```python
from build123d import *

# Parameters (mm, degrees)
BOSS_EXTRUDE1_DEPTH                               = 75
SKETCH5_R                                         = 1.75
CUT_EXTRUDE1_DEPTH                                = 2
CSK_FOR_0_FLAT_HEAD_MACHINE_SCREW_100_D           = 1.778
CSK_FOR_0_FLAT_HEAD_MACHINE_SCREW_100_DEPTH       = 3.302
CSK_FOR_0_FLAT_HEAD_MACHINE_SCREW_100_CSINK_D     = 3.0226
CSK_FOR_0_FLAT_HEAD_MACHINE_SCREW_100_CSINK_ANGLE = 100
CSK_FOR_0_FLAT_HEAD_MACHINE_SCREW_100_TIP         = 0.53416509
CHAMFER1_SIZE                                     = 3
BOSS_EXTRUDE2_DEPTH                               = 5
CHAMFER2_SIZE                                     = 3
CSK_FOR_0_FLAT_HEAD_MACHINE_SCREW_2_D             = 1.778
CSK_FOR_0_FLAT_HEAD_MACHINE_SCREW_2_DEPTH         = 3.302
CSK_FOR_0_FLAT_HEAD_MACHINE_SCREW_2_CSINK_D       = 3.0226
CSK_FOR_0_FLAT_HEAD_MACHINE_SCREW_2_CSINK_ANGLE   = 100
CSK_FOR_0_FLAT_HEAD_MACHINE_SCREW_2_TIP           = 0.53416509


with BuildPart() as part:
    # Sketch1 → Boss-Extrude1 (new body)
    with BuildSketch(Plane.XY):
        Polygon((-2, -3), (2, -3), (2, -0.5), (0, -0.5), (0, 0.5), (2, 0.5), (2, 3), (-2, 3), align=None)
    extrude(amount=BOSS_EXTRUDE1_DEPTH)

    # Sketch5 → Cut-Extrude1 (cut)
    with BuildSketch(Plane(origin=(2, 0, 0), x_dir=(0, 0, -1), z_dir=(1, 0, 0))):
        with Locations((-65, 0)):
            Circle(SKETCH5_R)
        with Locations((-46.66667, 0)):
            Circle(SKETCH5_R)
        with Locations((-28.33334, 0)):
            Circle(SKETCH5_R)
        with Locations((-10.00001, 0)):
            Circle(SKETCH5_R)
    extrude(amount=-CUT_EXTRUDE1_DEPTH, mode=Mode.SUBTRACT)

    # CSK for _0 Flat Head Machine Screw _100
    with Locations(Plane(origin=(0, 0, 0), x_dir=(0, 0, -1), z_dir=(1, 0, 0))):
        with Locations((-65, 0), (-10.00001, 0), (-46.66667, 0), (-28.33334, 0)):
            CounterSinkHole(CSK_FOR_0_FLAT_HEAD_MACHINE_SCREW_100_D / 2, CSK_FOR_0_FLAT_HEAD_MACHINE_SCREW_100_CSINK_D / 2, depth=CSK_FOR_0_FLAT_HEAD_MACHINE_SCREW_100_DEPTH, counter_sink_angle=CSK_FOR_0_FLAT_HEAD_MACHINE_SCREW_100_CSINK_ANGLE)
            with Locations((0, 0, -(CSK_FOR_0_FLAT_HEAD_MACHINE_SCREW_100_DEPTH + CSK_FOR_0_FLAT_HEAD_MACHINE_SCREW_100_TIP / 2))):  # 118° drill point
                Cone(0, CSK_FOR_0_FLAT_HEAD_MACHINE_SCREW_100_D / 2, CSK_FOR_0_FLAT_HEAD_MACHINE_SCREW_100_TIP, mode=Mode.SUBTRACT)

    # Chamfer1
    # the kernel refuses this chamfer: 3 mm, written as the material it takes off along each edge
    with BuildSketch(Plane(origin=(2, -3, -7.715048964), x_dir=(-0.9996219169112968, -0.027495876610586348, 0), z_dir=(0, 0, 1))) as chamfer1_piece_1:
        Polygon((CHAMFER1_SIZE * 0.999621916911, -CHAMFER1_SIZE * 0.0274958766106), (-CHAMFER1_SIZE * 0.0274958766106, -CHAMFER1_SIZE * 0.999621916911), (0, 0), align=None)
    extrude(amount=90.430097928, mode=Mode.SUBTRACT)
    with BuildSketch(Plane(origin=(2, 3, -7.715048964), x_dir=(-0.9996219169112968, 0.027495876610586348, 0), z_dir=(0, 0, 1))) as chamfer1_piece_2:
        Polygon((CHAMFER1_SIZE * 0.999621916911, CHAMFER1_SIZE * 0.0274958766106), (-CHAMFER1_SIZE * 0.0274958766106, CHAMFER1_SIZE * 0.999621916911), (0, 0), align=None)
    extrude(amount=90.430097928, mode=Mode.SUBTRACT)

    # Sketch6 → Boss-Extrude2 (add)
    with BuildSketch(Plane.XY.offset(75)):
        Polygon((0.5, 8), (3, 8), (3, 0.5), (0, 0.5), (0, -0.5), (2, -0.5), (2, -3), (-2, -3), (-2, 3), (0.5, 3), align=None)
    extrude(amount=BOSS_EXTRUDE2_DEPTH)

    # Chamfer2
    # the kernel refuses this chamfer: 3 mm, written as the material it takes off along each edge
    with BuildSketch(Plane(origin=(2, -3, 67.284951036), x_dir=(-0.9996219169112968, -0.027495876610586348, 0), z_dir=(0, 0, 1))) as chamfer2_piece_1:
        Polygon((CHAMFER2_SIZE * 0.999621916911, -CHAMFER2_SIZE * 0.0274958766106), (-CHAMFER2_SIZE * 0.0274958766106, -CHAMFER2_SIZE * 0.999621916911), (0, 0), align=None)
    extrude(amount=20.430097928, mode=Mode.SUBTRACT)

    # CSK for _0 Flat Head Machine Screw _ 2
    with Locations(Plane(origin=(3, 0, 0), x_dir=(0, 0, -1), z_dir=(1, 0, 0))):
        with Locations((-77.5, 5.5)):
            CounterSinkHole(CSK_FOR_0_FLAT_HEAD_MACHINE_SCREW_2_D / 2, CSK_FOR_0_FLAT_HEAD_MACHINE_SCREW_2_CSINK_D / 2, depth=CSK_FOR_0_FLAT_HEAD_MACHINE_SCREW_2_DEPTH, counter_sink_angle=CSK_FOR_0_FLAT_HEAD_MACHINE_SCREW_2_CSINK_ANGLE)
            with Locations((0, 0, -(CSK_FOR_0_FLAT_HEAD_MACHINE_SCREW_2_DEPTH + CSK_FOR_0_FLAT_HEAD_MACHINE_SCREW_2_TIP / 2))):  # 118° drill point
                Cone(0, CSK_FOR_0_FLAT_HEAD_MACHINE_SCREW_2_D / 2, CSK_FOR_0_FLAT_HEAD_MACHINE_SCREW_2_TIP, mode=Mode.SUBTRACT)


solid = part.part
```
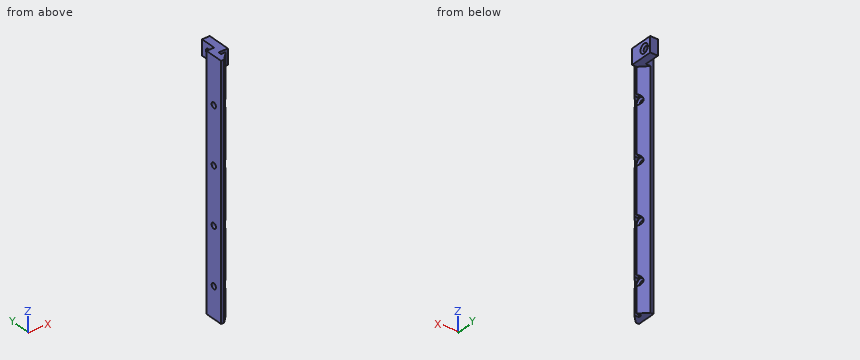
The model under review builds one solid part; all positions refer to its coordinate system, in mm. Round coordinates to 2 decimals unless told otherwise and drop trailing zeros. Loops run counter-clockwise (first coordinate to the right, second up) from the corner with the lowest first, then second, coordinate; pieces in that order, holes last. Notation, with made-up numbers: M -14.75,63 L 22.25,63 A9 cw 22.25,70 Z; hole C -5,28 d4. An arc over 180 degrees is marked long. Write item = value, one per line.
Item 1: Take a section at A-A on z = 77.5. Write out the cut boundary in (x, y), then the cut area to 3 significant figures.
Return value:
outline = M -2,-3 L -1,-3 L 1.5,-0.5 L 0,-0.5 L 0,0.5 L 3,0.5 L 3,3.99 L 2.48,4.61 L 0.5,4.61 L 0.5,3 L -2,3 Z; M 0.5,6.39 L 2.48,6.39 L 3,7.01 L 3,8 L 0.5,8 Z
area = 27.9 mm2
Item 2: Take a section at B-B on z = 13. Write out the cut boundary in (x, y).
Return value:
outline = M -2,-3 L -1,-3 L 1.5,-0.5 L 0,-0.5 L 0,0.5 L 1.5,0.5 L -1,3 L -2,3 Z
Item 3: For line 1 (Z direction, x = -1.25, y = 0); line 2 (X direction, y = 0.25, z = 55); line 3 (Z direction, x = 0.7, y = 6.5), list the stretches that pass through material, from the lowest coordinate up. Write a range as [from, to].
Return value:
line_1 = [0, 9.11], [10.89, 27.44], [29.22, 45.78], [47.56, 64.11], [65.89, 80]
line_2 = [-2, 0]
line_3 = [75, 80]
Item 4: Take a section at C-C on z = 65. Write out the cut boundary in (x, y).
Return value:
outline = M -2,-3 L -1,-3 L 0.25,-1.75 L 0,-1.75 L 0,-1.51 L -0.52,-0.89 L -2,-0.89 Z; M -2,0.89 L -0.52,0.89 L 0,1.51 L 0,1.75 L 0.25,1.75 L -1,3 L -2,3 Z
Item 5: Insertion check: P1, Ø1.8, axis at y = 0.5, z = 37.5, coming from the +X side; P2, Ø0.8, axis at x = 0.5, z = 55.5, coming from the -Y side; P3, Ø0.8, axis at x = -1, z = 52.5, coming from the +Y side; P4, Ø2, axis at y = 5, z = 60, coming from the -X side. Each pin has a flat end and moves straight along its axis. Give the tip position at first contact, or say it passes through.
Return value:
P1 = 1.5
P2 = -1.9
P3 = 3
P4 = through
